```python
from build123d import *

# Parameters (mm, degrees)
F0_R         = 1.75
F1_DEPTH     = 6
F0_R_2       = 19
F2_DEPTH     = 26
F3_T1_DEPTH  = 51.0048285071
F3_T3_DEPTH  = 32.5024142536
F3_T5_DEPTH  = 23.67798751
F3_T7_DEPTH  = 31.0048285071
F3_T9_DEPTH  = 43.67798751
F3_T11_DEPTH = 28.3837127694


# Not quite as in the source:
# - a fillet or chamfer that OpenCascade refuses, or shapes differently, is made with other operations: its cross-section is extruded or revolved along the edge and cut away or added


with BuildPart() as f1:
    # F0 (on Top) → F1 (new body)
    with BuildSketch(Plane.XY):
        with BuildLine():
            Line((-47.9554124177, 37.5), (-54.25, 37.5))
            add(Edge.make_bspline(
                [(-68.25, 30), (-54.25, 30), (-54.25, 37.5)],
                knots=[1.5707963268, 1.5707963268, 1.5707963268, 3.1415926536, 3.1415926536, 3.1415926536], degree=2, weights=[1, 0.7071067812, 1]))
            Line((-68.25, 30), (-68.25, -22.5))
            Line((-68.25, -22.5), (-47.9554124177, -22.5))
            Line((-47.9554124177, -22.5), (-47.9554124177, 37.5))
        make_face()
        with Locations((-55.2723892033, -14)):
            Circle(F0_R, mode=Mode.SUBTRACT)
        with Locations((-55.2723892033, 13.9999985695)):
            Circle(F0_R, mode=Mode.SUBTRACT)
        with Locations((-55.2723892033, 28.9999985695)):
            Circle(F0_R, mode=Mode.SUBTRACT)
        with BuildLine():
            Line((-68.25, -22.5), (-68.25, 30))
            add(Edge.make_bspline(
                [(-75.25, 31.0048094716), (-72.001288694, 30), (-68.25, 30)],
                knots=[1.0471975512, 1.0471975512, 1.0471975512, 1.5707963268, 1.5707963268, 1.5707963268], degree=2, weights=[1, 0.9659258263, 1]))
            Line((-75.25, 31.0048094716), (-75.25, 30))
            Line((-75.25, 30), (-75.25, -22.5))
            Line((-75.25, -22.5), (-68.25, -22.5))
        make_face()
    extrude(amount=-F1_DEPTH)

    # F0 (on Top) → F2 (join)
    with BuildSketch(Plane.XY):
        with BuildLine():
            add(Edge.make_bspline(
                [(-82.25, 37.5), (-82.25, 33.1698729811), (-75.25, 31.0048094716)],
                knots=[0, 0, 0, 1.0471975512, 1.0471975512, 1.0471975512], degree=2, weights=[1, 0.8660254038, 1]))
            Line((-82.25, 37.5), (-105.25, 37.5))
            ThreePointArc((-105.25, 37.5), (-126.4632034356, 28.7132034356), (-135.25, 7.5))
            Line((-135.25, 7.5), (-135.25, -22.5))
            Line((-135.25, -22.5), (-75.25, -22.5))
            Line((-75.25, -22.5), (-75.25, 30))
            Line((-75.25, 30), (-75.25, 31.0048094716))
        make_face()
        with Locations((-125.4025432638, -12.6525432638)):
            Circle(F0_R, mode=Mode.SUBTRACT)
        with Locations((-105.25, 7.5)):
            Circle(F0_R_2, mode=Mode.SUBTRACT)
        with Locations((-85.0974567362, 27.6525432638)):
            Circle(F0_R, mode=Mode.SUBTRACT)
    extrude(amount=-F2_DEPTH)

    # F3: fillet of radius 5 on 8 edges, made by hand

    # F3_s2 → F3_t1 (cut)
    with BuildSketch(Plane.XY.offset(-38.5024142536)):
        with BuildLine():
            ThreePointArc((-130.2490343146, -22.5004), (-133.7855339059, -21.0355339059), (-135.2504, -17.4990343146))
            Line((-135.2504, -17.4990343146), (-135.7505365685, -17.4990343146))
            ThreePointArc((-135.7505365685, -17.4990343146), (-135.7501365685, -19.9995171573), (-135.7501365685, -22.5))
            Line((-135.7501365685, -22.5), (-135.25, -23.0001365685))
            ThreePointArc((-135.25, -23.0001365685), (-132.7495171573, -23.0001365685), (-130.2490343146, -23.0005365685))
            Line((-130.2490343146, -23.0005365685), (-130.2490343146, -22.5004))
        make_face()
    extrude(amount=F3_T1_DEPTH, mode=Mode.SUBTRACT)

    # F3_s4 → F3_t3 (cut)
    with BuildSketch(Plane.XY.offset(-38.5024142536)):
        with BuildLine():
            ThreePointArc((-80.2509656854, -22.5004), (-76.7144660941, -21.0355339059), (-75.2496, -17.4990343146))
            Line((-75.2496, -17.4990343146), (-74.7494634315, -17.4990343146))
            ThreePointArc((-74.7494634315, -17.4990343146), (-74.7498634315, -19.9995171573), (-74.7498634315, -22.5))
            Line((-74.7498634315, -22.5), (-75.25, -23.0001365685))
            ThreePointArc((-75.25, -23.0001365685), (-77.7504828427, -23.0001365685), (-80.2509656854, -23.0005365685))
            Line((-80.2509656854, -23.0005365685), (-80.2509656854, -22.5004))
        make_face()
    extrude(amount=F3_T3_DEPTH, mode=Mode.SUBTRACT)

    # F3_s6 → F3_t5 (cut)
    with BuildSketch(Plane.XY.offset(-14.838993755)):
        with BuildLine():
            ThreePointArc((-50.7144025206, 37.5004), (-53.1463779594, 36.8692922228), (-54.9645855955, 35.1352441979))
            Line((-54.9645855955, 35.1352441979), (-55.389603903, 35.3988651863))
            ThreePointArc((-55.389603903, 35.3988651863), (-54.9183796159, 36.414502766), (-54.7501365685, 37.5))
            Line((-54.7501365685, 37.5), (-54.25, 38.0001365685))
            ThreePointArc((-54.25, 38.0001365685), (-52.4822012603, 38.0001365685), (-50.7144025206, 38.0005365685))
            Line((-50.7144025206, 38.0005365685), (-50.7144025206, 37.5004))
        make_face()
    extrude(amount=F3_T5_DEPTH, mode=Mode.SUBTRACT)

    # F3_s8 → F3_t7 (cut)
    with BuildSketch(Plane.XY.offset(-18.5024142536)):
        with BuildLine():
            ThreePointArc((-52.9563781031, 37.5004), (-49.4198785117, 36.0355339059), (-47.9550124177, 32.4990343146))
            Line((-47.9550124177, 32.4990343146), (-47.4548758491, 32.4990343146))
            ThreePointArc((-47.4548758491, 32.4990343146), (-47.4552758491, 34.9995171573), (-47.4552758491, 37.5))
            Line((-47.4552758491, 37.5), (-47.9554124177, 38.0001365685))
            ThreePointArc((-47.9554124177, 38.0001365685), (-50.4558952604, 38.0001365685), (-52.9563781031, 38.0005365685))
            Line((-52.9563781031, 38.0005365685), (-52.9563781031, 37.5004))
        make_face()
        with BuildLine():
            ThreePointArc((-52.9563781031, -22.5004), (-49.4198785117, -21.0355339059), (-47.9550124177, -17.4990343146))
            Line((-47.9550124177, -17.4990343146), (-47.4548758491, -17.4990343146))
            ThreePointArc((-47.4548758491, -17.4990343146), (-47.4552758491, -19.9995171573), (-47.4552758491, -22.5))
            Line((-47.4552758491, -22.5), (-47.9554124177, -23.0001365685))
            ThreePointArc((-47.9554124177, -23.0001365685), (-50.4558952604, -23.0001365685), (-52.9563781031, -23.0005365685))
            Line((-52.9563781031, -23.0005365685), (-52.9563781031, -22.5004))
        make_face()
    extrude(amount=F3_T7_DEPTH, mode=Mode.SUBTRACT)

    # F3_s10 → F3_t9 (cut)
    with BuildSketch(Plane.XY.offset(-34.838993755)):
        with BuildLine():
            ThreePointArc((-81.5354144045, 35.1352441979), (-83.3536220406, 36.8692922228), (-85.7855974794, 37.5004))
            Line((-85.7855974794, 37.5004), (-85.7855974794, 38.0005365685))
            ThreePointArc((-85.7855974794, 38.0005365685), (-84.0177987397, 38.0001365685), (-82.25, 38.0001365685))
            Line((-82.25, 38.0001365685), (-81.7498634315, 37.5))
            ThreePointArc((-81.7498634315, 37.5), (-81.5816203841, 36.414502766), (-81.110396097, 35.3988651863))
            Line((-81.110396097, 35.3988651863), (-81.5354144045, 35.1352441979))
        make_face()
    extrude(amount=F3_T9_DEPTH, mode=Mode.SUBTRACT)

    # F3_s12 → F3_t11 (cut)
    with BuildSketch(Plane.XY.offset(-34.3837127694)):
        with BuildLine():
            ThreePointArc((-77.9590299164, 32.0970407857), (-75.9803326171, 30.2544669483), (-75.2496, 27.6513243877))
            Line((-75.2496, 27.6513243877), (-74.7493950565, 27.6513243877))
            ThreePointArc((-74.7493950565, 27.6513243877), (-74.7497950565, 29.3280669297), (-74.7497950565, 31.0048094716))
            Line((-74.7497950565, 31.0048094716), (-75.1021974152, 31.4826790996))
            ThreePointArc((-75.1021974152, 31.4826790996), (-76.4425248665, 31.9557259843), (-77.7297679646, 32.5416124255))
            Line((-77.7297679646, 32.5416124255), (-77.9590299164, 32.0970407857))
        make_face()
    extrude(amount=F3_T11_DEPTH, mode=Mode.SUBTRACT)


solid = f1.part
```
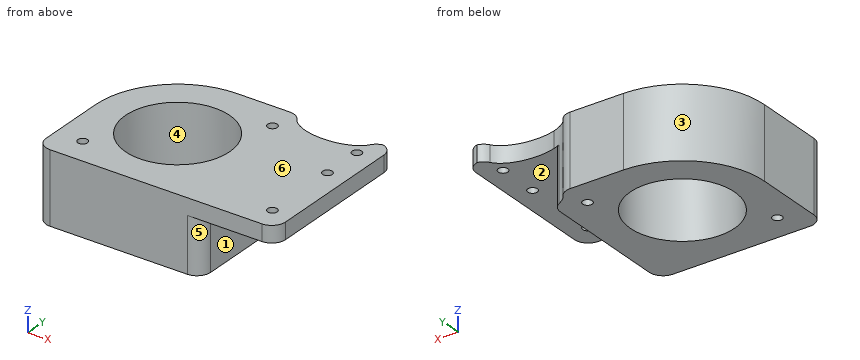
For this review, take the finished solid that the model builds, in its own axes (mm). Face numbers are marked on the shaded views. A direction names the side the tool comes from. Round coordinates to 2 decimals unless told otherwise and drop trailing zeros. Write each loop counter-clockwise with the first axis right and the second up, starting at its lowest first coordinate (ties: lowest second). Pieces come first, ordered by that corner, then holes. Notation, with made-up numbers: (28.25, 51) - (58.25, 51) arc R21 ccw to (58.25, 60) - close; hole circle Ø10 at (62.5, 87.5). An arc over 180 degrees is marked (long way). Answer as a JSON object with one key per item and string values.
1. We need section A-A on y = 1. Give the boundary of the cut face in (x, z), then the cut area to 3 significant figures.
Response values:
{"outline": "(-135.25, -26) - (-123.1, -26) - (-123.1, 0) - (-135.25, 0) - close; (-87.4, -26) - (-75.25, -26) - (-75.25, -6) - (-47.96, -6) - (-47.96, 0) - (-87.4, 0) - close", "area": "795 mm2"}
2. Draft analysis for pull direction X (two halves, no side actions). For the marked faces 1, 2, 3 and 4, state which applies: +X half, -X half, draft (parallel to the pull), parting line (faces both ways), or undercut.
Response values:
{"face 1": "+X half", "face 2": "draft", "face 3": "-X half", "face 4": "undercut"}
3. We need section C-C on z = -8. Count the separate pieces of the cut face and the enclosed holes in it, then the cut area to 3 significant figures.
Response values:
{"separate pieces": "1", "enclosed holes": "3", "area": "2,210 mm2"}
4. Tool access review of the marked faces 5 and 6: name each direction out of +Z, -Z, +X, -X, +Y, -Y from which nothing blocks a thin tool from reaching the whole face with its end or side.
Response values:
{"face 5": "-Z, +X, -Y", "face 6": "+Z, +X, -X, +Y, -Y"}
5. To check wall thickness, follow line 1 along Y through (x, z) = (-105.25, -13); line 2 along Z through (x, y) = (-63, -9.5); line 3 along Y through (x, z) = (-94.5, -6). State the ranges of each line that lie inside material, in increasing order.
Response values:
{"line 1": "y = -22.5 to -11.5, 26.5 to 37.5", "line 2": "z = -6 to 0", "line 3": "y = -22.5 to -8.17, 23.17 to 37.5"}
6. For pin 1 Ø4.5 at (x, y) = (-55.27, 29) entering from -Z; pin 2 Ø3 at (x, y) = (-55.27, 14) entering from +Z; pin 3 Ø8 at (y, z) = (12, -21) entering from -X; pin 4 Ø10 at (y, z) = (-6.5, -15) entering from +X, all flat-tipped, find the tip position at first contact; note any pin that passes through.
Response values:
{"pin 1": "stops at z = -6", "pin 2": "passes through", "pin 3": "stops at x = -135.25", "pin 4": "stops at x = -75.25"}
7. We need section D-D on x = -121. Give the boundary of the cut face in (y, z).
Response values:
{"outline": "(-22.5, -26) - (-3.13, -26) - (-3.13, 0) - (-22.5, 0) - close; (18.13, -26) - (33.03, -26) - (33.03, 0) - (18.13, 0) - close"}
8. We need section B-B on x = -99. Give the boundary of the cut face in (y, z).
Response values:
{"outline": "(-22.5, -26) - (-10.44, -26) - (-10.44, 0) - (-22.5, 0) - close; (25.44, -26) - (37.5, -26) - (37.5, 0) - (25.44, 0) - close"}
